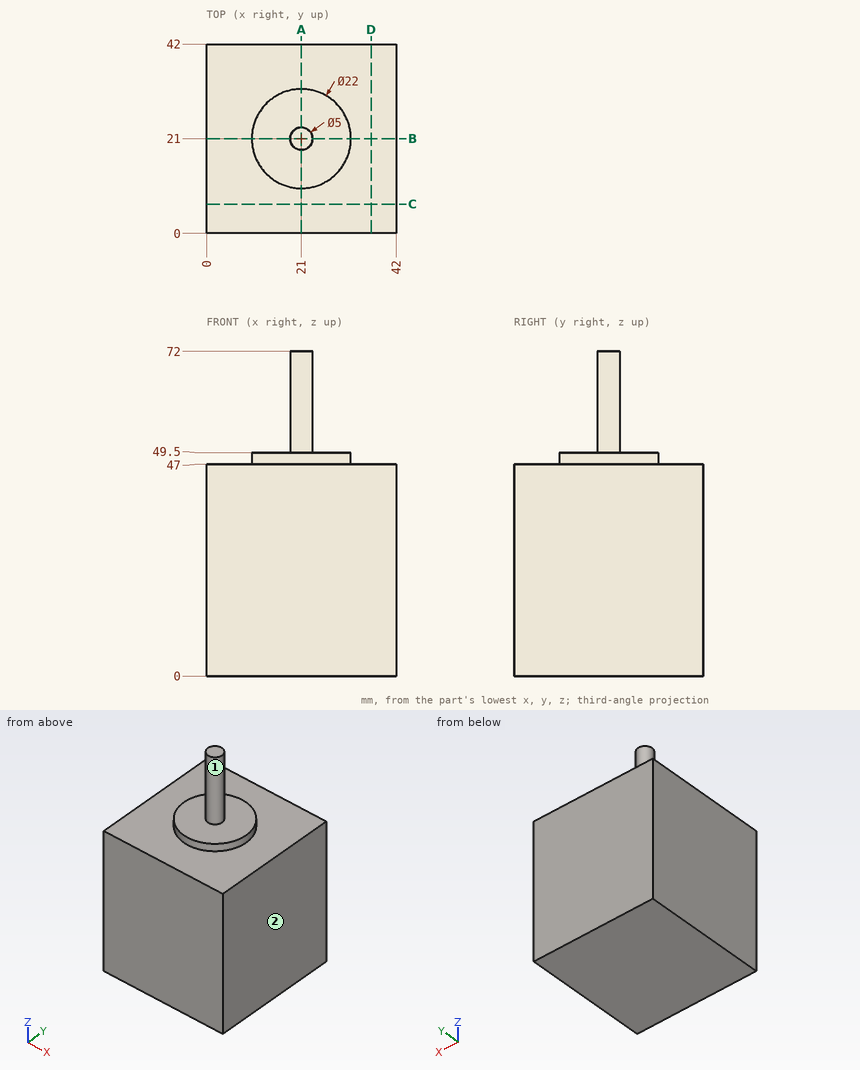
Design review of the part shown in the three views and the two pictorial views. Dimensions are in mm from the part's minimum x, y and z. A direction names the side the tool comes from. Coordinates: 2 decimals unless noted, no trailing zeros. Loops run counter-clockwise (first coordinate to the right, second up) from the corner with the lowest first, then second, coordinate; pieces in that order, holes last. Notation, with made-up numbers: (63.25, 33.25) - (85.25, 33.25) arc R25 ccw to (85.25, 64.25) - close; hole circle Ø3 at (75, 7.25). An arc over 180 degrees is marked (long way). Use a Markdown table: item, result. Add a question column.
Item 1: Insertion check: pin 1 Ø4 at (x, y) = (35, 37.5) entering from +Z; pin 2 Ø1.5 at (x, y) = (17.5, 23) entering from +Z; pin 3 Ø8 at (x, z) = (18, 57) entering from -Y. Each pin has a flat end and moves straight along its axis. Give the tip position at first contact, or say it passes through.
Item 2: We need section C-C (y = 6.5). Give the boundary of the cut face in (x, z), and give its area (3 significant figures).
Item 3: Tool access review of the marked faces 1 and 2: name each direction out of +Z, -Z, +X, -X, +Y, -Y from which nothing blocks a thin tool from reaching the whole face with its end or side.
Item 4: We need section A-A (x = 21). Give the boundary of the cut face in (y, z).
Item 5: For line 1 (Z direction, x = 24, y = 19); line 2 (Z direction, x = 26.5, y = 40.5); line 3 (Y direction, x = 20, z = 48.5), list the stretches that pass through material, from the lowest coordinate up.
Results list:
| question | item | result |
|---|---|---|
| 1 | pin 1 | stops at z = 47 |
| 1 | pin 2 | stops at z = 49.5 |
| 1 | pin 3 | stops at y = 18.5 |
| 2 | outline | (0, 0) - (42, 0) - (42, 47) - (0, 47) - close |
| 2 | area | 1,970 mm^2 |
| 3 | face 1 | +Z |
| 3 | face 2 | +Z, -Z, +X, +Y, -Y |
| 4 | outline | (0, 0) - (42, 0) - (42, 47) - (32, 47) - (32, 49.5) - (23.5, 49.5) - (23.5, 72) - (18.5, 72) - (18.5, 49.5) - (10, 49.5) - (10, 47) - (0, 47) - close |
| 5 | line 1 | z = 0 to 49.5 |
| 5 | line 2 | z = 0 to 47 |
| 5 | line 3 | y = 10.05 to 31.95 |
